The figure shows three views and two pictorial views of one solid part (mm, origin at its lowest corner). Answer the questions. A direction names the side the tool comes from. Coordinates: 2 decimals unless noted, no trailing zeros. Loops run counter-clockwise (first coordinate to the right, second up) from the corner with the lowest first, then second, coordinate; pieces in that order, holes last. Notation, with made-up numbers: M 72,62.5 L 127,62.5 A8 cw 127,66.5 Z; hole C -37.75,-13 d11. An arc over 180 degrees is marked long. Write each question's results on one line, items separated by ' | '.
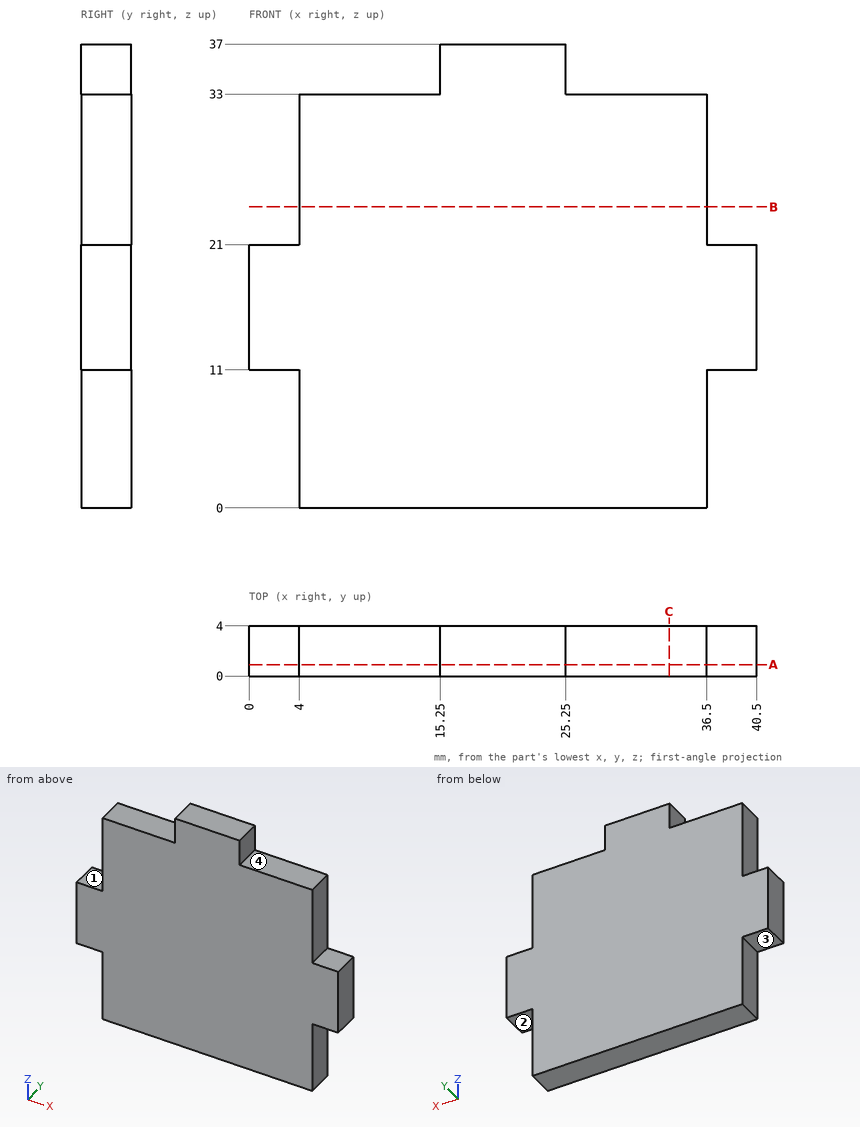
1) Find section C-C, the plane x = 33.5. Give the vertices of the cut face in (y, z), and give its area (3 significant figures).
Check result:
outline: M 0,0 L 4,0 L 4,33 L 0,33 Z | area: 132 mm^2
2) Which of the six approach directions +Z, -Z, +X, -X, +Y, -Y give full straight-line access (tool end or side, diameter ignored) to the marked faces 1, 2, 3 and 4?
Check result:
face 1: +Z, -X, +Y, -Y | face 2: -Z, +X, +Y, -Y | face 3: -Z, -X, +Y, -Y | face 4: +Z, +X, +Y, -Y
3) Find section A-A, the plane y = 0.9. Give the vertices of the cut face in (x, z), and give its area (3 significant figures).
Check result:
outline: M 0,11 L 4,11 L 4,0 L 36.5,0 L 36.5,11 L 40.5,11 L 40.5,21 L 36.5,21 L 36.5,33 L 25.25,33 L 25.25,37 L 15.25,37 L 15.25,33 L 4,33 L 4,21 L 0,21 Z | area: 1,190 mm^2
4) Straight lines are drawn through the part: probe 1 along Z at (x, y) = (26.5, 1.4); probe 2 along X at (y, z) = (0.6, 28.5); probe 3 along Z at (x, y) = (37, 3.55). For each, find the intervals that lie inside material, in ascending order. Write a range as [from, to].
Check result:
probe 1: [0, 33] | probe 2: [4, 36.5] | probe 3: [11, 21]
5) Find section B-B, the plane z = 24. Give the vertices of the cut face in (x, y), and give its area (3 significant figures).
Check result:
outline: M 4,0 L 36.5,0 L 36.5,4 L 4,4 Z | area: 130 mm^2
6) Given pin 1 Ø2 at (y, z) = (3, 6.5) entering from -X; pin 2 Ø1 at (x, y) = (6, 3.5) entering from +Z; pin 3 Ø1.2 at (x, y) = (38.5, 3) entering from -Z, each flat-ended and moving along its own axis, determine where each tip first touches the part or whether it passes through.
Check result:
pin 1: x = 4 | pin 2: z = 33 | pin 3: z = 11
